```python
from build123d import *

# Parameters (mm, degrees)
SKETCH1_R           = 2.15
BOSS_EXTRUDE1_DEPTH = 14
FILLET1_R           = 2


with BuildPart() as part:
    # Sketch1 → Boss-Extrude1 (new body)
    with BuildSketch(Plane.XY):
        with BuildLine():
            Line((-43.345, -10), (43.345, -10))
            ThreePointArc((43.345, -10), (53.345, 0), (43.345, 10))
            Line((43.345, 10), (-43.345, 10))
            ThreePointArc((-43.345, 10), (-53.345, 0), (-43.345, -10))
        make_face()
        with Locations((-43.345, 0)):
            Circle(SKETCH1_R, mode=Mode.SUBTRACT)
        with Locations((43.345, 0)):
            Circle(SKETCH1_R, mode=Mode.SUBTRACT)
    extrude(amount=BOSS_EXTRUDE1_DEPTH)

    # Fillet1
    fillet1_edges = [part.edges().sort_by_distance(p)[0] for p in [
        (-53.345, 0, 14),
        (0, -10, 14),
        (53.345, 0, 14),
        (0, -10, 0),
        (-53.345, 0, 0),
        (0, 10, 0),
        (53.345, 0, 0),
        (0, 10, 14),
    ]]
    fillet(fillet1_edges, radius=FILLET1_R)


solid = part.part
```
For this review, take the finished solid that the model builds, in its own axes (mm). Coordinates: 2 decimals unless noted, no trailing zeros. Write each loop counter-clockwise with the first axis right and the second up, starting at its lowest first coordinate (ties: lowest second). Pieces come first, ordered by that corner, then holes. Notation, with made-up numbers: (62, 3.25) - (111, 3.25) arc R29 ccw to (111, 35.25) - close; hole circle Ø9 at (76.5, -12.75). An arc over 180 degrees is marked (long way). Answer in a Markdown table with one row per item. Add a question column.
Q1. We need section B-B, the plane z = 10.75. State the section outline as (x, y) points (3 decimals).
Q2. For probe 1 along X at (y, z) = (-1.75, 13); probe 2 along Y at (x, z) = (-45, 7.75); probe 3 along Y at (x, z) = (-34, 12.25), list the stretches that pass through material, from the lowest coordinate up.
Q3. For P1, Ø5, axis at y = 5.5, z = 11.5, coming from the -X side; P2, Ø10, axis at x = -20, y = 0.5, coming from the -Z side; P3, Ø4, axis at y = 6, z = 2.5, coming from the +X side, all flat-tipped, find the tip position at first contact; note any pin that passes through.
Q4. Draft analysis for pull direction X (two halves, no side actions). For faces 1 (the cylindrical face through (-53.343, 0.22, 6.93)), 2 (the cylindrical face through (-44.93, 1.45, 6.9)), 3 (the flat face through (1, 10, 7)), state which applies: +X half, -X half, draft (parallel to the pull), parting line (faces both ways), or undercut.
Q5. We need section A-A, the plane y = 0. State the section outline as (x, z) points (3 decimals).
Answer list:
| question | item | result |
|---|---|---|
| 1 | outline | (-43.345, -10) - (43.345, -10) arc R10 ccw to (43.345, 10) - (-43.345, 10) arc R10 ccw to start; hole circle Ø4.3 at (-43.345, 0); hole circle Ø4.3 at (43.345, 0) |
| 2 | probe 1 | x = -52.92 to -44.59, -42.1 to 42.1, 44.59 to 52.92 |
| 2 | probe 2 | y = -9.86 to -1.37, 1.37 to 9.86 |
| 2 | probe 3 | y = -9.98 to 9.98 |
| 3 | P1 | stops at x = -52.88 |
| 3 | P2 | stops at z = 0 |
| 3 | P3 | stops at x = 52.51 |
| 4 | face 1 | -X half |
| 4 | face 2 | undercut |
| 4 | face 3 | draft |
| 5 | outline | (-53.345, 2) arc R2 ccw to (-51.345, 0) - (-45.495, 0) - (-45.495, 14) - (-51.345, 14) arc R2 ccw to (-53.345, 12) - close; (-41.195, 0) - (41.195, 0) - (41.195, 14) - (-41.195, 14) - close; (45.495, 0) - (51.345, 0) arc R2 ccw to (53.345, 2) - (53.345, 12) arc R2 ccw to (51.345, 14) - (45.495, 14) - close |
